Autodesk Inventor part; units mm, degrees
ref_plane "YZ Plane" through (0, 0, 0) normal (1, 0, 0) x (0, 1, 0)
ref_plane "XZ Plane" through (0, 0, 0) normal (0, 1, 0) x (-1, 0, 0)
ref_plane "XY Plane" through (0, 0, 0) normal (0, 0, 1) x (1, 0, 0)
sketch "Sketch1" plane through (0, 0, 0) normal (0, 0, 1) x (1, 0, 0)
  line L0 (0, 0) -> (0, 50.8)
  line L1 (0, 50.8) -> (3.175, 50.8)
  line L2 (3.175, 50.8) -> (3.175, 3.175)
  line L3 (3.175, 3.175) -> (50.8, 3.175)
  line L4 (50.8, 3.175) -> (50.8, 0)
  line L5 (50.8, 0) -> (0, 0)
  dimension "d0" = 50.8
  dimension "d1" = 3.175
  dimension "d4" = 50.8
extrude "Extrusion1" add sketch "Sketch1" along normal blind 1143
hole "Hole1" at (25.4, 3.175, 1104.9) direction (0, -1, 0) diameter 6.731 depth 25.4 tip angle 118
pattern_linear "Rectangular Pattern1" count 4 spacing 355.6 along (0, 0, -1) of "Hole1"
hole "Hole2" at (3.175, 25.4, 1104.9) direction (-1, 0, 0) diameter 6.731 depth 25.4 tip angle 118
pattern_linear "Rectangular Pattern2" count 4 spacing 355.6 along (0, 0, -1) of "Hole2", "Hole1"
properties part number "GE-12063"
The listing builds one solid part. Answer for the finished solid, in the listing's coordinates (mm). A direction names the side the tool comes from. Coordinates: 2 decimals unless noted, no trailing zeros. Order: outer loops, then holes, each group sorted by start corner. A loop starts at its lowest first (then second) coordinate and runs counter-clockwise, first axis right, second up. Notation, with made-up numbers: (6, 28.25) -> (48, 28.25) arc R31 cw to (48, 63.25) -> close; hole circle Ø10 at (3, 5). An arc over 180 degrees is marked (long way). Answer in a Markdown table with one row per item. Add a question column.
Item 1: Find the intervals of material crossed by L1, parallel to Z at x = 25.4, y = 0.9; L2, parallel to Z at x = 25, y = 1; L3, parallel to Y at x = 1.3, z = 1104.9, in increasing order. Write a range as from..to.
Item 2: Which of the six approach directions +Z, -Z, +X, -X, +Y, -Y give full straight-line access (tool end or side, diameter ignored) to faces 1 (the face through (3.175, 27, 563)), 2 (the face through (26, 0, 563))?
Item 3: Find section A-A (z = 475.5). Write down the section's boundary in (x, y) (3 decimals), then the cut area to 4 significant figures.
Item 4: Each of these flat-tipped pins is pushed along its axis until it touches: P1, Ø1.5, axis at x = 19.5, z = 162, coming from the +Y side (3 decimals); P2, Ø8, axis at y = 45.5, z = 874, coming from the +X side (3 decimals). Where does it stop, or does it pass through?
Result set:
| question | item | result |
|---|---|---|
| 1 | L1 | z = 0..34.73, 41.47..390.33, 397.07..745.93, 752.67..1101.53, 1108.27..1143 |
| 1 | L2 | z = 0..34.76, 41.44..390.36, 397.04..745.96, 752.64..1101.56, 1108.24..1143 |
| 1 | L3 | y = 0..22.03, 28.77..50.8 |
| 2 | face 1 | +Z, -Z, +X, +Y |
| 2 | face 2 | +Z, -Z, +X, -X, -Y |
| 3 | outline | (0, 0) -> (50.8, 0) -> (50.8, 3.175) -> (3.175, 3.175) -> (3.175, 50.8) -> (0, 50.8) -> close |
| 3 | area | 312.5 mm² |
| 4 | P1 | stops at y = 3.175 |
| 4 | P2 | stops at x = 3.175 |
